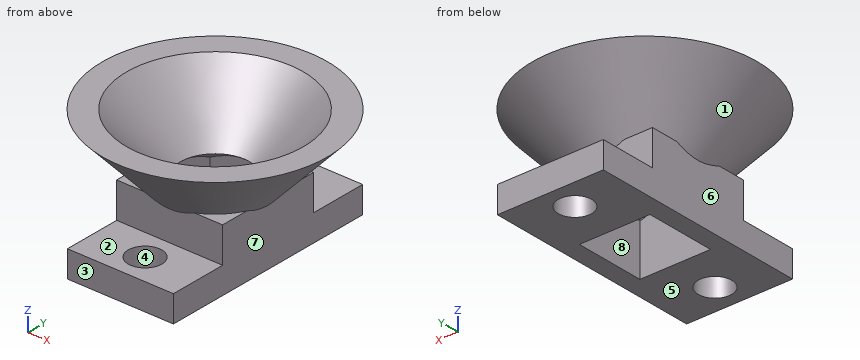
from build123d import *

# Parameters (mm, degrees)
F0_W     = 12
F0_H     = 25
F0_R     = 1.9
F0_W_2   = 8
F0_H_2   = 8
F1_DEPTH = 3
F2_W     = 12
F2_H     = 12
F2_W_2   = 8
F2_H_2   = 8
F3_DEPTH = 4


with BuildPart() as f1:
    # F0 (on Top) → F1 (new body)
    with BuildSketch(Plane.XY):
        Rectangle(F0_W, F0_H)
        with Locations((0, -9.25)):
            Circle(F0_R, mode=Mode.SUBTRACT)
        Rectangle(F0_W_2, F0_H_2, mode=Mode.SUBTRACT)
        with Locations((0, 9.25)):
            Circle(F0_R, mode=Mode.SUBTRACT)
    extrude(amount=F1_DEPTH)

    # F2 (on face) → F3 (join)
    with BuildSketch(Plane.XY.offset(3)):
        Rectangle(F2_W, F2_H)
        Rectangle(F2_W_2, F2_H_2, mode=Mode.SUBTRACT)
    extrude(amount=F3_DEPTH)

    # F5 (on Right) → F6 (revolve)
    with BuildSketch(Plane.YZ):
        Polygon((3.891662, 7.005772), (5.491862, 5.790449), (12.732967, 13.621861), (10.009052, 13.621861), align=None)
    revolve(axis=Axis((0, 0, 7.370598), (0, 0, -1)))


solid = f1.part
The listing builds one solid part. Answer for the finished solid, in the listing's coordinates (mm). Face numbers are marked on the shaded views. A direction names the side the tool comes from. Give positions to 0.01 mm unless a question says otherwise; leave off trailing zeros. Loops run counter-clockwise (first coordinate to the right, second up) from the corner with the lowest first, then second, coordinate; pieces in that order, holes last. Notation, with made-up numbers: (59.25, 75.25) - (92.25, 75.25) arc R35 cw to (92.25, 113.25) - close; hole circle Ø5 at (-7, -17.5). An arc over 180 degrees is marked (long way). Answer as a JSON object with one key per item and string values.
1. A cutting plane is placed at A-A (y = 0). Write down the section's boundary in (x, z), then the cut area to 3 significant figures.
Determined:
{"outline": "(-12.73, 13.62) - (-6, 6.34) - (-6, 0) - (-4, 0) - (-4, 6.92) - (-3.89, 7.01) - (-10.01, 13.62) - close; (3.89, 7.01) - (4, 6.92) - (4, 0) - (6, 0) - (6, 6.34) - (12.73, 13.62) - (10.01, 13.62) - close", "area": "64.5 mm²"}
2. A cutting plane is placed at B-B (x = 0). Write down the section's boundary in (y, z), then the cut area to 3 significant figures.
Determined:
{"outline": "(-12.73, 13.62) - (-6, 6.34) - (-6, 3) - (-7.35, 3) - (-7.35, 0) - (-4, 0) - (-4, 6.92) - (-3.89, 7.01) - (-10.01, 13.62) - close; (-12.5, 0) - (-11.15, 0) - (-11.15, 3) - (-12.5, 3) - close; (3.89, 7.01) - (4, 6.92) - (4, 0) - (7.35, 0) - (7.35, 3) - (6, 3) - (6, 6.34) - (12.73, 13.62) - (10.01, 13.62) - close; (11.15, 0) - (12.5, 0) - (12.5, 3) - (11.15, 3) - close", "area": "80.7 mm²"}
3. For the marked faces 1, 2, 3 and 4, determine the directions among +Z, -Z, +X, -X, +Y, -Y from which every point of the face is accessible in a straight line to the end or side of a thin tool.
Determined:
{"face 1": "none", "face 2": "+X, -X, -Y", "face 3": "-Z, +X, -X, -Y", "face 4": "-Z"}
4. Find the intervals of material crossed by L1, parallel to Y at x = 0, z = 0.9; L2, parallel to X at y = 1, z = 5.75; L3, parallel to Z at x = -5.75, y = -9.75, in increasing order. Write a range as [from, to].
Determined:
{"L1": "[-12.5, -11.15], [-7.35, -4], [4, 7.35], [11.15, 12.5]", "L2": "[-6, -4], [4, 6]", "L3": "[0, 3], [12.09, 13.62]"}
5. Flat-ended cylindrical pins translate along their axes: pin 1 Ø1 at (x, y) = (4, -3.5) entering from +Z; pin 2 Ø1.2 at (x, z) = (-0.5, 4.5) entering from -Y; pin 3 Ø1.5 at (x, y) = (-8, 3) entering from +Z. Find the tip coordinate at first contact, or state that the pin passes through.
Determined:
{"pin 1": "z = 9.09", "pin 2": "y = -6", "pin 3": "z = 12.85"}
6. A cutting plane is placed at C-C (z = 10.25). Write down the section's boundary in (x, y), then the cut area to 3 significant figures.
Determined:
{"outline": "circle Ø19.23 at (0, 0); hole circle Ø13.78 at (0, 0)", "area": "141 mm²"}
7. A cutting plane is placed at D-D (y = -9.25). Give the number of separate pieces and of enclosed holes in the cut face, then the cut area to 3 significant figures.
Determined:
{"separate pieces": "3", "enclosed holes": "0", "area": "63.0 mm²"}
8. For a pull along X with two mould halves and no side action, classify the marked faces 5, 6, 7 and 8 as pulls with the +X half, pulls with the -X half, needs draft (parallel to the pull), parting line crosses it, or undercut.
Determined:
{"face 5": "needs draft", "face 6": "pulls with the -X half", "face 7": "pulls with the +X half", "face 8": "undercut"}
